```python
from build123d import *

# Parameters (mm, degrees)
F0_W     = 38.1
F0_H     = 38.1
F0_W_2   = 32.004
F0_H_2   = 32.004
F1_DEPTH = 330.2
F2_R     = 15.875
F2_R_2   = 12.827
F3_DEPTH = 152.4
F4_R     = 3.175
F5_DEPTH = 38.101


with BuildPart() as f1:
    # F0 (on Front) → F1 (new body)
    with BuildSketch(Plane.XZ):
        Rectangle(F0_W, F0_H)
        Rectangle(F0_W_2, F0_H_2, mode=Mode.SUBTRACT)
    extrude(amount=F1_DEPTH)

    # F2 (on face) → F3 (join)
    with BuildSketch(Plane.YZ.offset(19.05)):
        with Locations((-304.8, 0)):
            Circle(F2_R)
        with Locations((-304.8, 0)):
            Circle(F2_R_2, mode=Mode.SUBTRACT)
    extrude(amount=F3_DEPTH)

    # F4 (on face) → F5 (cut, through all)
    with BuildSketch(Plane.YZ.offset(19.05)):
        with Locations((-19.05, 0)):
            Circle(F4_R)
    extrude(amount=-F5_DEPTH, mode=Mode.SUBTRACT)


solid = f1.part
```
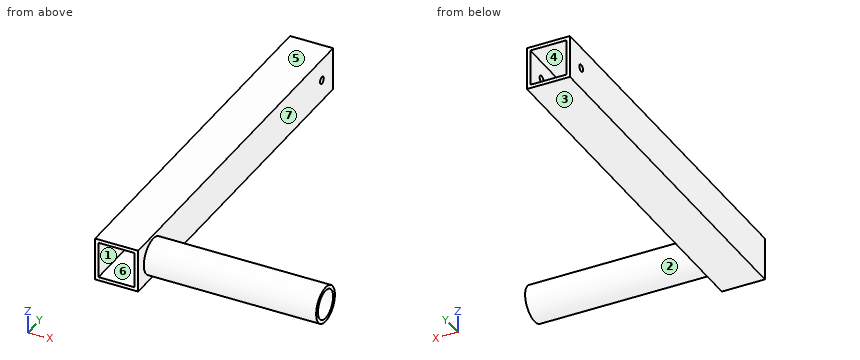
Source: CAD feature listing. Evaluate the final solid. Frame: model axes, mm. Face numbers are marked on the shaded views. A direction names the side the tool comes from. Give positions to 0.01 mm unless a question says otherwise; leave off trailing zeros. Write each loop counter-clockwise with the first axis right and the second up, starting at its lowest first coordinate (ties: lowest second). Pieces come first, ordered by that corner, then holes.
1. Section query C-C (x = 5.5). Return the cut outline in (y, z), then the cut area to 3 significant figures.
2. Access query for the marked faces 1, 2 and 3. Directions: +Z, -Z, +X, -X, +Y, -Y. A direction counts if a zero-diameter tool reaches every point of the face in a straight line with its end or side. Return the directions, or none.
3. Section query A-A (z = 0). Return the cut outline in (x, y) (3 decimals), then the cut area to 3 significant figures.
4. Section query B-B (y = -19.05). Return the cut outline in (x, z) (3 decimals), then the cut area to 3 significant figures.
5. First-contact query: pin 1 (3 mm diameter, centred on x = 140, z = 9, fed in from -Y); pin 2 (9.5 mm diameter, centred on y = -211.5, z = -1, fed in from +X); pin 3 (5.5 mm diameter, centred on y = -19.05, z = 0, fed in from +X); pin 4 (1.5 mm diameter, centred on x = 34, z = -1, fed in from +Y). Flat tips, straight axial feed; report the tip coordinate or a pass-through.
6. Pull-direction query (X, two-part tool) for the marked faces 4, 5, 6 and 7; classes: +X half, -X half, draft (parallel to the pull), parting line (faces both ways), or undercut.
7. Material intervals for line 1 along X through (y, z) = (-200, 9); line 2 along Z through (x, y) = (-16.65, -19.05) (3 decimals), sorted ascending.
8. Section query D-D (y = -304.8). Return the cut outline in (x, z) (3 decimals).
Output values:
1. outline: (-330.2, -19.05) - (0, -19.05) - (0, -16) - (-330.2, -16) - close; (-330.2, 16) - (0, 16) - (0, 19.05) - (-330.2, 19.05) - close
1. area: 2,010 mm2
2. face 1: +Y, -Y
2. face 2: +X
2. face 3: -Z, +X, -X, +Y, -Y
3. outline: (-19.05, -330.2) - (-16.002, -330.2) - (-16.002, -22.225) - (-19.05, -22.225) - close; (-19.05, -15.875) - (-16.002, -15.875) - (-16.002, 0) - (-19.05, 0) - close; (16.002, -330.2) - (19.05, -330.2) - (19.05, -320.675) - (171.45, -320.675) - (171.45, -317.627) - (19.05, -317.627) - (19.05, -291.973) - (171.45, -291.973) - (171.45, -288.925) - (19.05, -288.925) - (19.05, -22.225) - (16.002, -22.225) - close; (16.002, -15.875) - (19.05, -15.875) - (19.05, 0) - (16.002, 0) - close
3. area: 2,900 mm2
4. outline: (-19.05, -19.05) - (19.05, -19.05) - (19.05, -3.175) - (16.002, -3.175) - (16.002, -16.002) - (-16.002, -16.002) - (-16.002, -3.175) - (-19.05, -3.175) - close; (-19.05, 3.175) - (-16.002, 3.175) - (-16.002, 16.002) - (16.002, 16.002) - (16.002, 3.175) - (19.05, 3.175) - (19.05, 19.05) - (-19.05, 19.05) - close
4. area: 389 mm2
5. pin 1: stops at y = -318.79
5. pin 2: stops at x = 19.05
5. pin 3: passes through
5. pin 4: stops at y = -288.93
6. face 4: undercut
6. face 5: draft
6. face 6: undercut
6. face 7: +X half
7. line 1: x = -19.05 to -16, 16 to 19.05
7. line 2: z = -19.05 to -3.175, 3.175 to 19.05
8. outline: (-19.05, -19.05) - (19.05, -19.05) - (19.05, -15.875) - (171.45, -15.875) - (171.45, -12.827) - (19.05, -12.827) - (19.05, 12.827) - (171.45, 12.827) - (171.45, 15.875) - (19.05, 15.875) - (19.05, 19.05) - (-19.05, 19.05) - close; hole (-16.002, -16.002) - (16.002, -16.002) - (16.002, 16.002) - (-16.002, 16.002) - close
